```python
from build123d import *

# Parameters (mm, degrees)
SKETCH1_R           = 2.2
BOSS_EXTRUDE1_DEPTH = 1


with BuildPart() as part:
    # Sketch1 → Boss-Extrude1 (new body)
    with BuildSketch(Plane(origin=(0, 0, 0), x_dir=(1, 0, 0), z_dir=(0, 1, 0))):
        Polygon((0, -39.5), (3, -39.5), (3, -41.5), (0, -41.5), (0, -105), (58, -105), (58, -41.5), (55, -41.5), (55, -39.5), (58, -39.5), (108, -39.5), (108, 39.5), (58, 39.5), (55, 39.5), (55, 41.5), (58, 41.5), (58, 105), (0, 105), (0, 41.5), (3, 41.5), (3, 39.5), (0, 39.5), (-50, 39.5), (-50, -39.5), align=None)
        with Locations(Location((4, 97.5, 0), (0, 0, 270))):
            Circle(SKETCH1_R, mode=Mode.SUBTRACT)
        with Locations(Location((54, 97.5, 0), (0, 0, 270))):
            Circle(SKETCH1_R, mode=Mode.SUBTRACT)
        with Locations(Location((54, 47.5, 0), (0, 0, 270))):
            Circle(SKETCH1_R, mode=Mode.SUBTRACT)
        with Locations(Location((4, 47.5, 0), (0, 0, 270))):
            Circle(SKETCH1_R, mode=Mode.SUBTRACT)
        with Locations(Location((4, -47.5, 0), (0, 0, 270))):
            Circle(SKETCH1_R, mode=Mode.SUBTRACT)
        with Locations(Location((54, -47.5, 0), (0, 0, 270))):
            Circle(SKETCH1_R, mode=Mode.SUBTRACT)
        with Locations(Location((54, -97.5, 0), (0, 0, 270))):
            Circle(SKETCH1_R, mode=Mode.SUBTRACT)
        with Locations(Location((4, -97.5, 0), (0, 0, 270))):
            Circle(SKETCH1_R, mode=Mode.SUBTRACT)
        with Locations(Location((-40, 30, 0), (0, 0, 270))):
            Circle(SKETCH1_R, mode=Mode.SUBTRACT)
        with Locations(Location((-10, 30, 0), (0, 0, 270))):
            Circle(SKETCH1_R, mode=Mode.SUBTRACT)
        with Locations(Location((-40, -30, 0), (0, 0, 270))):
            Circle(SKETCH1_R, mode=Mode.SUBTRACT)
        with Locations(Location((-10, -30, 0), (0, 0, 270))):
            Circle(SKETCH1_R, mode=Mode.SUBTRACT)
        with Locations(Location((68, -30, 0), (0, 0, 270))):
            Circle(SKETCH1_R, mode=Mode.SUBTRACT)
        with Locations(Location((98, -30, 0), (0, 0, 270))):
            Circle(SKETCH1_R, mode=Mode.SUBTRACT)
        with Locations(Location((98, 30, 0), (0, 0, 270))):
            Circle(SKETCH1_R, mode=Mode.SUBTRACT)
        with Locations(Location((68, 30, 0), (0, 0, 270))):
            Circle(SKETCH1_R, mode=Mode.SUBTRACT)
    extrude(amount=BOSS_EXTRUDE1_DEPTH)


solid = part.part
```
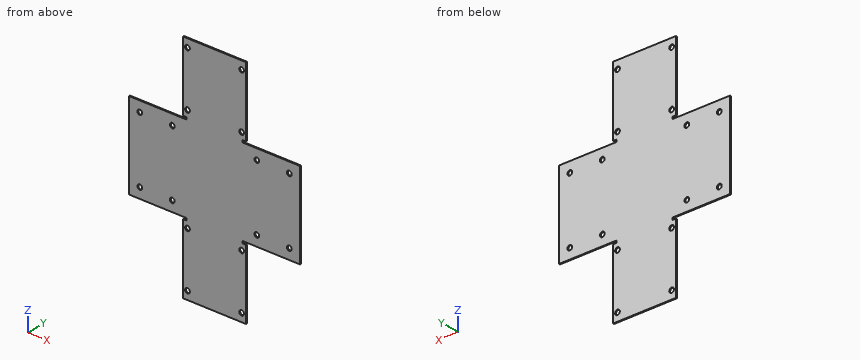
The model under review builds one solid part; all positions refer to its coordinate system, in mm. Round coordinates to 2 decimals unless told otherwise and drop trailing zeros. Loops run counter-clockwise (first coordinate to the right, second up) from the corner with the lowest first, then second, coordinate; pieces in that order, holes last. Notation, with made-up numbers: M 76.25,75 L 85.25,75 A37 ccw 85.25,112 Z; hole C -7,16.25 d2. An arc over 180 degrees is marked long. Put each result on its own line as item: value.
Q1. To check wall thickness, follow L1, parallel to X at y = 0.7, z = 30; L2, parallel to X at y = 0.65, z = -97.5; L3, parallel to Z at x = -41.5, y = 0.4. State the ranges of each line that lie inside material, in increasing order.
Result set:
L1: x = -50 to -42.2, -37.8 to -12.2, -7.8 to 65.8, 70.2 to 95.8, 100.2 to 108
L2: x = 0 to 1.8, 6.2 to 51.8, 56.2 to 58
L3: z = -39.5 to -31.61, -28.39 to 28.39, 31.61 to 39.5
Q2. Consider section B-B, the plane z = 47.5. Give the boundary of the cut face in (x, y).
Result set:
outline: M 0,0 L 1.8,0 L 1.8,1 L 0,1 Z; M 6.2,0 L 51.8,0 L 51.8,1 L 6.2,1 Z; M 56.2,0 L 58,0 L 58,1 L 56.2,1 Z
Q3. Consider section D-D, the plane z = -79.5. Give the boundary of the cut face in (x, y).
Result set:
outline: M 0,0 L 58,0 L 58,1 L 0,1 Z
Q4. For pin 1 (0.5 mm diameter, centred on y = 0.5, z = 40.5, fed in from -X); pin 2 (4 mm diameter, centred on x = -10, z = 30, fed in from +Y); pin 3 (0.5 mm diameter, centred on y = 0.5, z = 88.5, fed in from +X), all flat-tipped, find the tip position at first contact; note any pin that passes through.
Result set:
pin 1: stops at x = 3
pin 2: passes through
pin 3: stops at x = 58
Q5. Consider section C-C, the plane y = 0.3. Count the separate pieces of the cut face and the enclosed holes in it, then the cut area to 3 significant figures.
Result set:
separate pieces: 1
enclosed holes: 16
area: 19,800 mm²
Q6. Consider section A-A, the plane x = 98. Give the boundary of the cut face in (y, z).
Result set:
outline: M 0,-39.5 L 1,-39.5 L 1,-32.2 L 0,-32.2 Z; M 0,-27.8 L 1,-27.8 L 1,27.8 L 0,27.8 Z; M 0,32.2 L 1,32.2 L 1,39.5 L 0,39.5 Z
